Verification items for the finished model (mm, model axes). Face numbers are marked on the shaded views. A direction names the side the tool comes from. Round coordinates to 2 decimals unless told otherwise and drop trailing zeros. Write each loop counter-clockwise with the first axis right and the second up, starting at its lowest first coordinate (ties: lowest second). Pieces come first, ordered by that corner, then holes. Notation, with made-up numbers: (16, -23) - (31, -23) arc R10 cw to (31, -16) - close; hole circle Ø1 at (26.25, 25.25). An arc over 180 degrees is marked (long way). Answer as a JSON object with one key per item and string values.
```python
from build123d import *

# Parameters (mm, degrees)
F0_W     = 100
F0_H     = 85
F0_W_2   = 31
F0_H_2   = 74
F1_DEPTH = 25
F2_DEPTH = 5
F3_R     = 5
F4_R     = 2


with BuildPart() as f1:
    # F0 (on Top) → F1 (new body)
    with BuildSketch(Plane.XY):
        Rectangle(F0_W, F0_H)
        Rectangle(F0_W_2, F0_H_2, mode=Mode.SUBTRACT)
    extrude(amount=F1_DEPTH)

    # F0 (on Top) → F2 (join)
    with BuildSketch(Plane.XY):
        Rectangle(F0_W_2, F0_H_2)
    extrude(amount=F2_DEPTH)

    # F3
    f3_edges = [f1.edges().sort_by_distance(p)[0] for p in [
        (0, 42.5, 25),
        (-50, 0, 25),
        (0, -42.5, 25),
        (50, 0, 25),
    ]]
    fillet(f3_edges, radius=F3_R)

    # F4
    f4_edges = [f1.edges().sort_by_distance(p)[0] for p in [
        (-15.5, 0, 25),
        (15.5, 0, 25),
    ]]
    fillet(f4_edges, radius=F4_R)


solid = f1.part
```
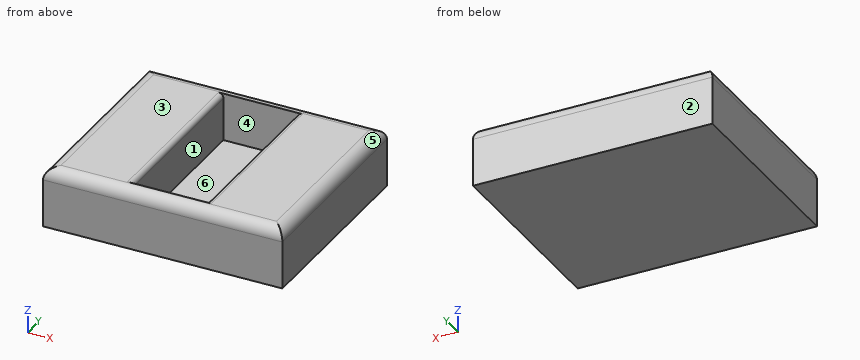
Q1. Material ranges on line 1 along X through (y, z) = (19.5, 12.5); line 2 along Y through (x, z) = (7, 17); line 3 along Z through (x, y) = (-13.5, 8), recorded low to high. Write a range as [from, to].
Geometry check:
{"line 1": "x = [-50, -15.5], [15.5, 50]", "line 2": "y = [-42.5, -37], [37, 42.5]", "line 3": "z = [0, 5]"}
Q2. Gauge pin test, flat end, axial feed: P1, Ø9.5, axis at x = 3.5, y = -11, coming from the +Z side. Record the tip position at first contact, or that the pin passes through.
Geometry check:
{"P1": "stops at z = 5"}
Q3. Section check A-A, the plane x = -6. Record the cut outline in (y, z).
Geometry check:
{"outline": "(-42.5, 0) - (42.5, 0) - (42.5, 20) arc R5 ccw to (37.5, 25) - (37, 25) - (37, 5) - (-37, 5) - (-37, 25) - (-37.5, 25) arc R5 ccw to (-42.5, 20) - close"}
Q4. Release check for a two-part mould opening along X. For the marked faces 3, 4, 5 and 6 record: released by +X, released by -X, zero draft, split by the parting line, or undercut.
Geometry check:
{"face 3": "zero draft", "face 4": "undercut", "face 5": "released by +X", "face 6": "undercut"}
Q5. Set-up check for the marked faces 1 and 2: record each of +Z, -Z, +X, -X, +Y, -Y from which the full face is reachable in a straight line by a thin tool's end or side.
Geometry check:
{"face 1": "+Z", "face 2": "+Z, -Z, +X, -X, +Y"}
Q6. Section check B-B, the plane z = 7.5. Record the cut outline in (x, y), then the cut area to 3 significant figures.
Geometry check:
{"outline": "(-50, -42.5) - (50, -42.5) - (50, 42.5) - (-50, 42.5) - close; hole (-15.5, -37) - (15.5, -37) - (15.5, 37) - (-15.5, 37) - close", "area": "6,210 mm2"}
Q7. Section check C-C, the plane y = 24.5. Record the cut outline in (x, z).
Geometry check:
{"outline": "(-50, 0) - (50, 0) - (50, 20) arc R5 ccw to (45, 25) - (17.5, 25) arc R2 ccw to (15.5, 23) - (15.5, 5) - (-15.5, 5) - (-15.5, 23) arc R2 ccw to (-17.5, 25) - (-45, 25) arc R5 ccw to (-50, 20) - close"}
